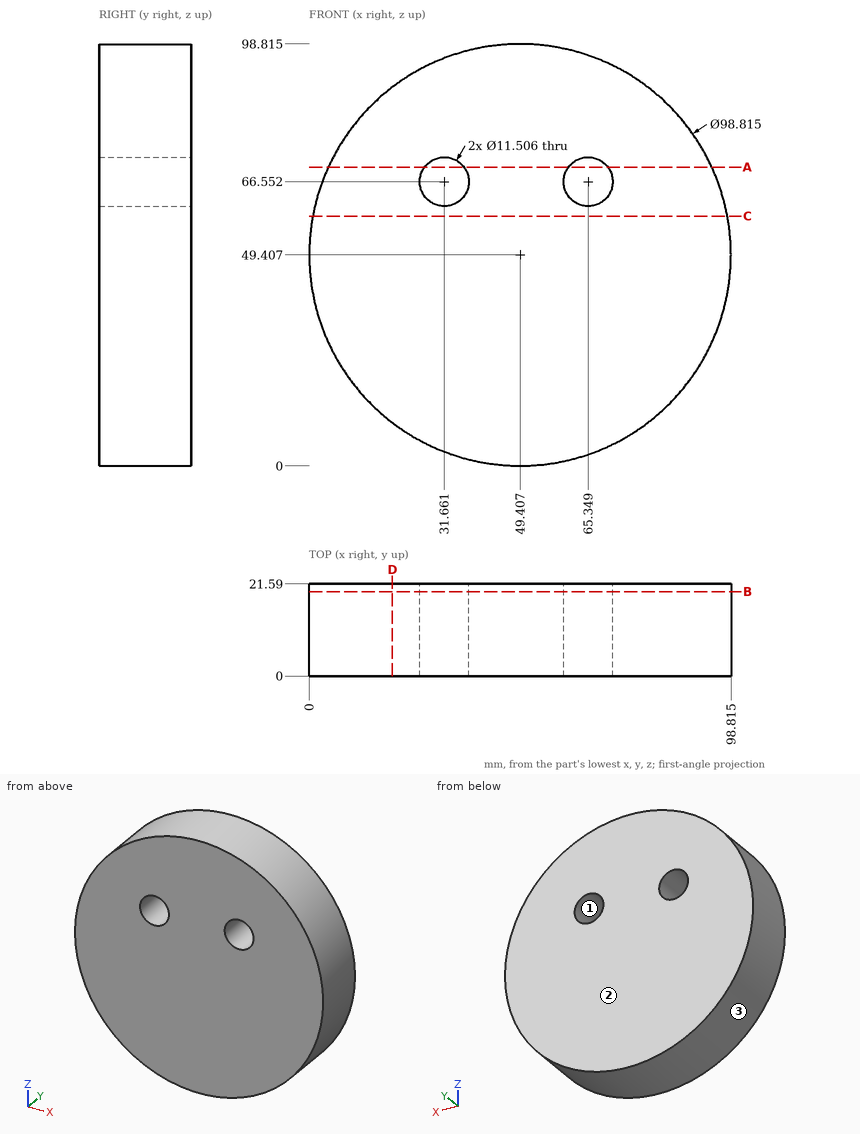
Study the drawing (mm; zero at the part's minimum x, y, z) and answer. Coordinates: 2 decimals unless noted, no trailing zeros. Loops run counter-clockwise (first coordinate to the right, second up) from the corner with the lowest first, then second, coordinate; pieces in that order, holes last. Notation, with made-up numbers: M 40,-4.5 L 56,-4.5 A35 ccw 56,34.5 Z; hole C 21,9.5 d9. An arc over 180 degrees is marked long. Answer in a Markdown table with one row per item.
1) Given pin 1 (1 mm diameter, centred on x = 16, y = 10.5, fed in from -Z) (1 decimal); pin 2 (3 mm diameter, centred on y = 9.5, z = 86.5, fed in from +X) (1 decimal); pin 3 (8 mm diameter, centred on x = 75.5, y = 5, fed in from +Z), each flat-ended and moving along its own axis, determine where each tip first touches the part or whether it passes through.
Answers below:
| item | result |
|---|---|
| pin 1 | z = 12.6 |
| pin 2 | x = 83.7 |
| pin 3 | z = 93.6 |
2) Find section C-C (z = 58.5). Determine the outline of the cut face in (x, y).
Answers below:
| item | result |
|---|---|
| outline | M 0.84,0 L 97.97,0 L 97.97,21.59 L 0.84,21.59 Z |
3) Find section D-D (x = 19.5). Determine the outline of the cut face in (y, z) (1 decimal), then the cut area to 3 significant figures.
Answers below:
| item | result |
|---|---|
| outline | M 0,10.1 L 21.6,10.1 L 21.6,88.7 L 0,88.7 Z |
| area | 1,700 mm^2 |
4) Determine the mould class of the marked faces 1, 2 and 3 for opening direction Z: released by +Z, released by -Z, zero draft, split by the parting line, or undercut.
Answers below:
| item | result |
|---|---|
| face 1 | undercut |
| face 2 | zero draft |
| face 3 | split by the parting line |
5) Find section B-B (y = 19.75). Determine the outline of the cut face in (x, z) (1 decimal).
Answers below:
| item | result |
|---|---|
| outline | C 49.4,49.4 d98.8; hole C 31.7,66.6 d11.5; hole C 65.3,66.6 d11.5 |
6) Find the intervals of material crossed by probe 1 along X at (y, z) = (17.25, 71.5) (1 decimal); probe 2 along Z at (x, y) = (30, 1.75) (1 decimal); probe 3 along Z at (x, y) = (61, 20.5) (1 decimal), in increasing order.
Answers below:
| item | result |
|---|---|
| probe 1 | 5.2 to 28.7, 34.6 to 62.4, 68.3 to 93.6 |
| probe 2 | 4 to 61, 72.1 to 94.8 |
| probe 3 | 1.4 to 62.8, 70.3 to 97.4 |
7) Find section A-A (z = 70). Determine the outline of the cut face in (x, y) (1 decimal), then the cut area to 3 significant figures.
Answers below:
| item | result |
|---|---|
| outline | M 4.5,0 L 27.1,0 L 27.1,21.6 L 4.5,21.6 Z; M 36.3,0 L 60.7,0 L 60.7,21.6 L 36.3,21.6 Z; M 70,0 L 94.3,0 L 94.3,21.6 L 70,21.6 Z |
| area | 1,540 mm^2 |
